The model under review builds one solid part; all positions refer to its coordinate system, in mm. Face numbers are marked on the shaded views. A direction names the side the tool comes from. Give positions to 0.01 mm unless a question says otherwise; leave off trailing zeros. Loops run counter-clockwise (first coordinate to the right, second up) from the corner with the lowest first, then second, coordinate; pieces in that order, holes last. Notation, with made-up numbers: M -38,58 L -31,58 A23 cw -31,69 Z; hole C 78.25,-20 d10. An arc over 180 degrees is marked long. Return JSON: item names as keys, results as strings.
```python
from build123d import *

# Parameters (mm, degrees)
F1_DEPTH = 63.5
F0_W     = 25.3858086348
F0_H     = 19.05
F2_DEPTH = 25.4
F3_DEPTH = 7.9375
F5_R     = 6.35
F7_D     = 6.35
F8_SIZE2 = 1.27
F8_SIZE  = 1.27


with BuildPart() as f1:
    # F0 (on Front) → F1 (new body, symmetric)
    with BuildSketch(Plane.XZ):
        Polygon((-41.275, 9.525), (-41.275, -9.525), (41.275, -9.525), (41.275, 9.525), (22.225, 9.525), align=None)
    extrude(amount=F1_DEPTH, both=True)

    # F0 (on Front) → F2 (join, symmetric)
    with BuildSketch(Plane.XZ):
        with Locations((73.0179043174, 52.4002)):
            Rectangle(F0_W, F0_H)
        with BuildLine():
            Line((22.225, 9.525), (41.275, 9.525))
            Line((41.275, 9.525), (41.275, 27.0002))
            ThreePointArc((41.275, 27.0002), (45.9246798487, 38.2255201513), (57.15, 42.8752))
            Line((57.15, 42.8752), (60.325, 42.8752))
            Line((60.325, 42.8752), (60.325, 61.9252))
            Line((60.325, 61.9252), (57.15, 61.9252))
            add(Edge.make_bspline(
                [(55.4113425633, 61.8818957059), (55.9890331624, 61.9003631029), (56.5685898657, 61.9148171773), (57.15, 61.9252)],
                knots=[110.1382061471, 110.1382061471, 110.1382061471, 110.1382061471, 111.5045361635, 111.5045361635, 111.5045361635, 111.5045361635], degree=3))
            ThreePointArc((55.4113425633, 61.8818957059), (31.8470531758, 51.073349088), (22.225, 27.0002))
            Line((22.225, 27.0002), (22.225, 9.525))
        make_face()
    extrude(amount=F2_DEPTH, both=True)

    # F0 (on Front) → F3 (join, symmetric)
    with BuildSketch(Plane.XZ):
        with BuildLine():
            add(Edge.make_bspline(
                [(-41.275, 9.525), (-25.5970072353, 32.826953112), (8.8444037337, 60.3932612228), (55.4113425633, 61.8818957059)],
                knots=[0, 0, 0, 0, 110.1382061471, 110.1382061471, 110.1382061471, 110.1382061471], degree=3))
            Line((-41.275, 9.525), (22.225, 9.525))
            Line((22.225, 9.525), (22.225, 27.0002))
            ThreePointArc((22.225, 27.0002), (31.8470531758, 51.073349088), (55.4113425633, 61.8818957059))
        make_face()
    extrude(amount=F3_DEPTH, both=True)

    # F0 (on Front) → F4 (revolve)
    with BuildSketch(Plane.XZ):
        Polygon((85.7108086348, 66.675), (85.7108086348, 61.9252), (85.7108086348, 42.8752), (85.7108086348, 38.1), (111.125, 38.1), (111.125, 66.675), align=None)
    revolve(axis=Axis((85.7108086348, 0, 52.3875), (0, 0, 1)))

    # F5
    f5_edges = [f1.edges().sort_by_distance(p)[0] for p in [
        (-41.275, -63.5, 0),
        (41.275, -63.5, 0),
        (41.275, 63.5, 0),
        (-41.275, 63.5, 0),
    ]]
    fillet(f5_edges, radius=F5_R)

    # F7 (through all)
    with Locations(Plane(origin=(0, 0, -9.525), x_dir=(1, 0, 0), z_dir=(0, 0, -1))):
        with Locations((-33.655, 55.88), (34.036, 55.88), (34.417, -56.134), (-33.274, -56.134)):
            Hole(F7_D / 2)

    # F8
    f8_edges = [f1.edges().sort_by_distance(p)[0] for p in [
        (60.296617, 0, 66.675),
    ]]
    chamfer(f8_edges, length=F8_SIZE, length2=F8_SIZE2)


solid = f1.part
```
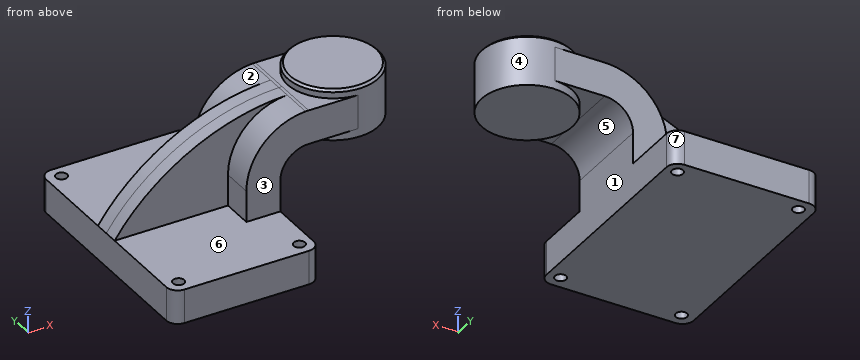
1) Tool access review of the marked faces 1, 2 and 3: name each direction out of +Z, -Z, +X, -X, +Y, -Y from which nothing blocks a thin tool from reaching the whole face with its end or side.
From the geometry:
{"face 1": "-Z, +X, +Y, -Y", "face 2": "+Z, -X, +Y", "face 3": "+Z, +X, -X, -Y"}
2) Insertion check: pin 1 (10 mm diameter, centred on x = 34.036, y = -55.88, fed in from +Z) (3 decimals); pin 2 (7.5 mm diameter, centred on x = 34.417, y = 56.134, fed in from -Z) (3 decimals); pin 3 (15 mm diameter, centred on x = 85.5, y = -9, fed in from -Z); pin 4 (1.5 mm diameter, centred on x = 93.5, z = 48, fed in from -Y). Each pin has a flat end and moves straight along its axis. Give the tip position at first contact, or say it passes through.
From the geometry:
{"pin 1": "z = 9.525", "pin 2": "z = -9.525", "pin 3": "z = 38.1", "pin 4": "y = -24.42"}
3) The part is to be moulded in two halves that separate along X. For the marked faces 4, 5, 6 and 7, say which applies: released by +X, released by -X, zero draft, split by the parting line, or undercut.
From the geometry:
{"face 4": "undercut", "face 5": "undercut", "face 6": "zero draft", "face 7": "released by +X"}
4) Consider section A-A on z = 5. Write out the cut boundary in (x, y) (3 decimals).
From the geometry:
{"outline": "M -41.275,-57.15 A6.35 ccw -34.925,-63.5 L 34.925,-63.5 A6.35 ccw 41.275,-57.15 L 41.275,57.15 A6.35 ccw 34.925,63.5 L -34.925,63.5 A6.35 ccw -41.275,57.15 Z; hole C -33.655,-55.88 d6.35; hole C -33.274,56.134 d6.35; hole C 34.036,-55.88 d6.35; hole C 34.417,56.134 d6.35"}
5) Consider section B-B on y = -33. Write out the cut boundary in (x, z) (3 decimals), then the cut area to 3 significant figures.
From the geometry:
{"outline": "M -41.275,-9.525 L 41.275,-9.525 L 41.275,9.525 L -41.275,9.525 Z", "area": "1,570 mm²"}
6) Wall thickness on L1, parallel to X at y = -55.88, z = 3 (3 decimals); L2, parallel to Y at x = -32, z = 0; L3, parallel to Z at x = 21, y = -9 (3 decimals): over which ranges is each line inside the solid? List them lowest first. Write a range as from..to.
From the geometry:
{"L1": "-41.275..-36.83, -30.48..30.861, 37.211..41.275", "L2": "-63.5..-58.59, -53.17..53.23, 59.04..63.5", "L3": "-9.525..9.525"}
